Verification items for the finished model (mm, model axes). Give positions to 0.01 mm unless a question says otherwise; leave off trailing zeros. Write each loop counter-clockwise with the first axis right and the second up, starting at its lowest first coordinate (ties: lowest second). Pieces come first, ordered by that corner, then holes. Notation, with made-up numbers: (-39, 10) -> (9, 10) arc R24 cw to (9, 22) -> close; hole circle Ø8 at (8.25, 60). An arc over 180 degrees is marked (long way). Write item = value, one per line.
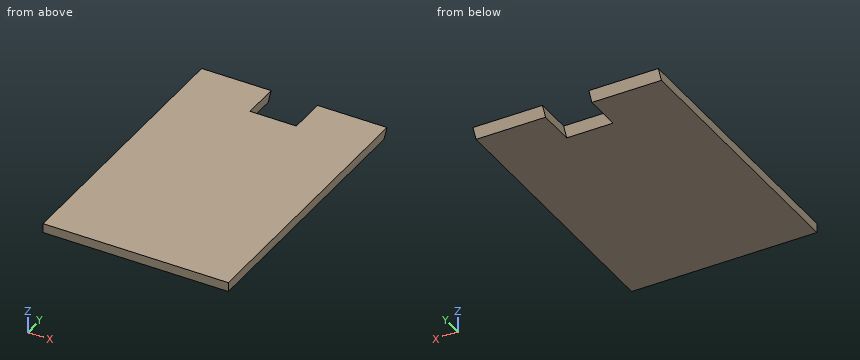
from build123d import *

# Parameters (mm, degrees)
BOSS_EXTRUDE1_DEPTH = 6.35
CUT_EXTRUDE1_DEPTH  = 31.75
CUT_EXTRUDE2_DEPTH  = 127


with BuildPart() as part:
    # Sketch1 → Boss-Extrude1 (new, symmetric)
    with BuildSketch(Plane.XY):
        Polygon((127, -190.5), (-127, -190.5), (-127, 190.5), (-31.75, 190.5), (-31.75, 139.7), (31.75, 139.7), (31.75, 190.5), (127, 190.5), align=None)
    extrude(amount=BOSS_EXTRUDE1_DEPTH, both=True)

    # Sketch4 → Cut-Extrude1 (cut, symmetric)
    with BuildSketch(Plane(origin=(0, 0, 0), x_dir=(0, 0, -1), z_dir=(1, 0, 0))):
        Polygon((-6.35, 139.7), (6.35, 139.7), (6.35, 132.367651581), align=None)
        Polygon((-6.35, 190.5), (6.35, 190.5), (6.35, 183.167651581), align=None)
    extrude(amount=CUT_EXTRUDE1_DEPTH, both=True, mode=Mode.SUBTRACT)

    # Sketch5 → Cut-Extrude2 (cut, symmetric)
    with BuildSketch(Plane(origin=(0, 0, 0), x_dir=(0, 0, -1), z_dir=(1, 0, 0))):
        Polygon((-6.35, 190.5), (6.35, 190.5), (6.35, 183.167651581), align=None)
    extrude(amount=CUT_EXTRUDE2_DEPTH, both=True, mode=Mode.SUBTRACT)


solid = part.part
Item 1: Sectioned sample at A-A on y = 164. Record the cut outline in (x, z), then the cut area to 3 significant figures.
Response values:
outline = (-127, -6.35) -> (-31.75, -6.35) -> (-31.75, 6.35) -> (-127, 6.35) -> close; (31.75, -6.35) -> (127, -6.35) -> (127, 6.35) -> (31.75, 6.35) -> close
area = 2,420 mm^2
Item 2: Sectioned sample at C-C on x = -15. Record the cut outline in (y, z), then the cut area to 3 significant figures.
Response values:
outline = (-190.5, -6.35) -> (132.37, -6.35) -> (139.7, 6.35) -> (-190.5, 6.35) -> close
area = 4,150 mm^2
Item 3: Sectioned sample at B-B on z = -2.5. Record the cut outline in (x, y).
Response values:
outline = (-127, -190.5) -> (127, -190.5) -> (127, 185.39) -> (31.75, 185.39) -> (31.75, 134.59) -> (-31.75, 134.59) -> (-31.75, 185.39) -> (-127, 185.39) -> close
Item 4: Material ranges on line 1 (Y direction, x = -40, z = 3.25); line 2 (Y direction, x = 86.5, z = 0.75), recorded low to high.
Response values:
line_1 = -190.5 to 188.71
line_2 = -190.5 to 187.27
Item 5: Go/stop test with a flat-tipped pin: P1, Ø6, axis at x = -28, z = -4.5, coming from the +Y side. Record where the tip stops, or that it passes through.
Response values:
P1 = 135.17
